from build123d import *

# Parameters (mm, degrees)
SKETCH1_R                    = 20.6375
SKETCH1_R_2                  = 5.159375
BASE_FLANGE1_DEPTH           = 6.35
EDGE_FLANGE1_STRIP_W         = 41.3004
EDGE_FLANGE1_STRIP_H         = 6.35
EDGE_FLANGE1_STRIP_CUT_DEPTH = 63.5
EDGE_FLANGE1_DEPTH           = 63.5
SKETCH9_R                    = 4.9609375
CUT_EXTRUDE1_DEPTH           = 184.910350528
CUT_EXTRUDE2_DEPTH           = 188.331726574
FILLET1_R                    = 19.05
FILLET2_R                    = 6.35
FILLET3_R                    = 12.7


# Sheet-metal steps are written as plain solids
with BuildPart() as part:
    # Sketch1 → Base-Flange1 (new body)
    with BuildSketch(Plane.XY):
        Polygon((0, 85.725), (31.75, 103.1875), (63.5, 85.725), (63.5, 0), (0, 0), align=None)
        with Locations((31.75, 60.96)):
            Circle(SKETCH1_R, mode=Mode.SUBTRACT)
        with Locations((31.75, 89.535)):
            Circle(SKETCH1_R_2, mode=Mode.SUBTRACT)
        with Locations((31.75, 32.385)):
            Circle(SKETCH1_R_2, mode=Mode.SUBTRACT)
    extrude(amount=-BASE_FLANGE1_DEPTH)

    # Edge-Flange1 strip (across the edge) → Edge-Flange1 strip cut (cut)
    with BuildSketch(Plane(origin=(63.5, 0, -6.35), x_dir=(0, 1, 0), z_dir=(-1, 0, 0))):
        with Locations((-6.35, -3.175)):
            Rectangle(EDGE_FLANGE1_STRIP_W, EDGE_FLANGE1_STRIP_H)
    extrude(amount=EDGE_FLANGE1_STRIP_CUT_DEPTH, mode=Mode.SUBTRACT)

    # Edge-Flange1 section (across the edge) → Edge-Flange1 (add)
    with BuildSketch(Plane(origin=(63.5, 0, -6.35), x_dir=(0, 1, 0), z_dir=(-1, 0, 0))):
        with BuildLine():
            Line((0, 7.9502), (0, 136.525))
            Line((0, 136.525), (6.35, 136.525))
            Line((6.35, 136.525), (6.35, 7.9502))
            ThreePointArc((6.35, 7.9502), (8.678559668, 2.328559668), (14.3002, 0))
            Line((14.3002, 0), (14.3002, -6.35))
            ThreePointArc((14.3002, -6.35), (4.188431608, -2.161568392), (0, 7.9502))
        make_face()
    extrude(amount=EDGE_FLANGE1_DEPTH)

    # Sketch9 → Cut-Extrude1 (cut, through all)
    with BuildSketch(Plane(origin=(0, 6.35, 0), x_dir=(1, 0, 0), z_dir=(0, 1, 0))):
        with Locations(Location((31.75, 30.226, 0), (0, 0, 270))):
            Circle(SKETCH9_R)
        with Locations(Location((31.75, 131.826, 0), (0, 0, 270))):
            Circle(SKETCH9_R)
    extrude(amount=-CUT_EXTRUDE1_DEPTH, mode=Mode.SUBTRACT)

    # Sketch10 → Cut-Extrude2 (cut, through all)
    with BuildSketch(Plane.XZ):
        Polygon((0, -142.875), (12.7, -142.875), (12.7, -93.6752), (0, -14.3002), align=None)
        Polygon((63.5, -142.875), (63.5, -14.3002), (50.8, -93.6752), (50.8, -142.875), align=None)
    extrude(amount=-CUT_EXTRUDE2_DEPTH, mode=Mode.SUBTRACT)

    # Fillet1
    fillet1_edges = [part.edges().sort_by_distance(p)[0] for p in [
        (31.75, 103.1875, -3.175),
    ]]
    fillet(fillet1_edges, radius=FILLET1_R)

    # Fillet2
    fillet2_edges = [part.edges().sort_by_distance(p)[0] for p in [
        (0, 85.725, -3.175),
        (63.5, 85.725, -3.175),
    ]]
    fillet(fillet2_edges, radius=FILLET2_R)

    # Fillet3
    fillet3_edges = [part.edges().sort_by_distance(p)[0] for p in [
        (50.8, 3.175, -142.875),
        (12.7, 3.175, -142.875),
    ]]
    fillet(fillet3_edges, radius=FILLET3_R)


solid = part.part
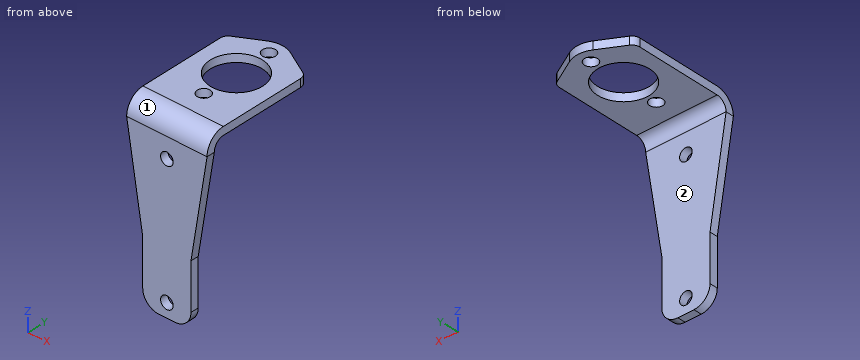
Design review of the part built by this model. Coordinates are the model's own, in mm. Face numbers are marked on the shaded views. A direction names the side the tool comes from. Give positions to 0.01 mm unless a question says otherwise; leave off trailing zeros. Loops run counter-clockwise (first coordinate to the right, second up) from the corner with the lowest first, then second, coordinate; pieces in that order, holes last. Notation, with made-up numbers: M -4.75,41 L 1.25,41 A21 ccw 1.25,60 Z; hole C 33,-13.75 d9. An arc over 180 degrees is marked long. One line per question, with ' | ' between items. Start each with the question number.
1. Add section A-A (y = 60.96). Write out the cut boundary in (x, z), plus the area to 3 significant figures.
2. Add section C-C (z = -27.5). Write out the cut boundary in (x, y), plus the area to 3 significant figures.
3. For the marked faces 1 and 2, list the 3-axis set-ups (+Z, -Z, +X, -X, +Y, -Y) from which the entire face can be reached by the end or side of a thin tool; tool diameter is ignored.
4. Insertion check: P1, Ø6, axis at x = 18.5, y = 78.5, coming from the -Z side; P2, Ø5, axis at y = 4, z = -115.5, coming from the +X side; P3, Ø1.9, axis at y = 3, z = -116.5, coming from the -X side; P4, Ø8.5, axis at x = 31.75, y = 89.535, coming from the -Z side. Each pin has a flat end and moves straight along its axis. Give the tip position at first contact, or say it passes through.
5. Add section B-B (x = 31.75). Give the number of separate pieces and of enclosed holes in the cut face, plus the area to 3 significant figures.
6. Add section D-D (x = 43). Write out the cut boundary in (y, z), plus the area to 3 significant figures.
7. To check wall thickness, follow L1, parallel to Y at x = 31, z = -4; L2, parallel to X at y = 60, z = -3; L3, parallel to Y at x = 39, z = -26.5. State the ranges of each line that lie inside material, in increasing order.
Worked out:
1) outline: M 0,-6.35 L 11.11,-6.35 L 11.11,0 L 0,0 Z; M 52.39,-6.35 L 63.5,-6.35 L 63.5,0 L 52.39,0 Z | area: 141 mm²
2) outline: M 2.11,0 L 27.61,0 L 27.61,6.35 L 2.11,6.35 Z; M 35.89,0 L 61.39,0 L 61.39,6.35 L 35.89,6.35 Z | area: 324 mm²
3) face 1: +Z, +X, -X, -Y | face 2: -Z, +X, -X, +Y
4) P1: stops at z = -6.35 | P2: stops at x = 50.8 | P3: stops at x = 12.7 | P4: passes through
5) separate pieces: 6 | enclosed holes: 0 | area: 956 mm²
6) outline: M 0,-141.89 L 6.35,-141.89 L 6.35,-14.3 A7.95 cw 14.3,-6.35 L 43.66,-6.35 L 43.66,0 L 14.3,0 A14.3 ccw 0,-14.3 Z; M 78.26,-6.35 L 97,-6.35 L 97,0 L 78.26,0 Z | area: 1,230 mm²
7) L1: y = 4.38 to 27.28, 37.49 to 40.34, 81.58 to 84.43, 94.64 to 100.48 | L2: x = 0 to 11.13, 52.37 to 63.5 | L3: y = 0 to 6.35
